Design review of the part built by this model. Coordinates are the model's own, in mm. A direction names the side the tool comes from. Coordinates: 2 decimals unless noted, no trailing zeros. Loops run counter-clockwise (first coordinate to the right, second up) from the corner with the lowest first, then second, coordinate; pieces in that order, holes last. Notation, with made-up numbers: M 45.5,87.5 L 55.5,87.5 A21 cw 55.5,116.5 Z; hole C 45.25,-16.75 d10. An arc over 180 degrees is marked long. Put each result on its own line as item: value. Start each with the question number.
(1) The part is to be moulded in two halves that separate along Z. For faces 4 (the flat face through (0, 0, -25)), 5 (the flat face through (-3, 12.5, 76)), 6 (the flat face through (-67, 0, 25)), say which applies: +Z half, -Z half, draft (parallel to the pull), parting line (faces both ways), or undercut.
(2) Take a section at D-D, the plane y = -27.5. Give the boundary of the cut face in (x, z).
(3) Take a section at A-A, the plane z = -100. Give the boundary of the cut face in (x, y).
(4) For probe 1 along Z at (x, y) = (69.5, 29); probe 2 along Y at (x, z) = (-16.5, 12); probe 3 along X at (y, z) = (13.5, -50), list the stretches that pass through material, from the lowest coordinate up. Write a range as [from, to].
(5) Clearance check with flat-ended pins moving along their axes: pin 1 (15 mm diameter, centred on y = 5.5, z = 9.5, fed in from +X); pin 2 (1.5 mm diameter, centred on x = -4, y = -8.5, fed in from -Z); pin 3 (12 mm diameter, centred on x = 3, z = 63, fed in from +Y). State where each tip first meets the part, or that it passes through.
(6) Take a section at B-B, the plane x = -65.5. Give the boundary of the cut face in (y, z).
(7) For faces 1 (the flat face through (-3, -22.5, -78)), 2 (the flat face through (67, 0, 25)), 3 (the flat face through (0, 0, 25)), list the 3-axis set-ups (+Z, -Z, +X, -X, +Y, -Y) from which the entire face can be reached by the end or side of a thin tool; tool diameter is ignored.
```python
from build123d import *

# Parameters (mm, degrees)
SKETCH1_W                = 175
SKETCH1_H                = 65
BOSS_EXTRUDE1_DEPTH      = 2
SKETCH2_W                = 175
SKETCH2_H                = 65
BOSS_EXTRUDE2_DEPTH      = 2
BOSS_EXTRUDE3_DEPTH      = 127
BOSS_EXTRUDE3_DEPTH_BACK = 127
SKETCH3_W                = 40
SKETCH3_H                = 4
BOSS_EXTRUDE4_DEPTH      = 2
BOSS_EXTRUDE5_DEPTH      = 2


with BuildPart() as part:
    # Sketch1 → Boss-Extrude1 (new body)
    with BuildSketch(Plane.XY.offset(25.0000008)):
        Rectangle(SKETCH1_W, SKETCH1_H)
    extrude(amount=BOSS_EXTRUDE1_DEPTH)



with BuildPart() as body_2:
    # Sketch2 → Boss-Extrude2 (new body)
    with BuildSketch(Plane.XY.offset(-25)):
        Rectangle(SKETCH2_W, SKETCH2_H)
    extrude(amount=-BOSS_EXTRUDE2_DEPTH)


with BuildPart() as part_1:
    add(part.part)

    add(body_2.part)  # Boss-Extrude3 merges body 2
    # Sketch3 → Boss-Extrude3 (add, two sides: drawn at the far end of the back side and taken through both)
    with BuildSketch(Plane.XY.offset(-BOSS_EXTRUDE3_DEPTH_BACK)):
        with Locations((-2.5, 14.5)):
            Rectangle(SKETCH3_W, SKETCH3_H)
        with Locations((-2.5, -20.5)):
            Rectangle(SKETCH3_W, SKETCH3_H)
    extrude(amount=BOSS_EXTRUDE3_DEPTH + BOSS_EXTRUDE3_DEPTH_BACK)

    # Sketch4 → Boss-Extrude4 (add)
    with BuildSketch(Plane(origin=(45.00000144, 0, 0), x_dir=(0, 0, -1), z_dir=(1, 0, 0))):
        Polygon((3.748957701, 32.5), (25, 32.5), (25, -32.5), (-25.0000008, -32.5), (-25.0000008, 32.5), (-3.748958501, 32.5), (-3.748958501, 25.45800753), (3.748957701, 25.45800753), align=None)
    extrude(amount=BOSS_EXTRUDE4_DEPTH)

    # Sketch5 → Boss-Extrude5 (add)
    with BuildSketch(Plane(origin=(-45.00000144, 0, 0), x_dir=(0, 0, -1), z_dir=(1, 0, 0))):
        Polygon((-25.0000008, 32.5), (-25.0000008, -32.5), (25, -32.5), (25, 32.5), (3.748957701, 32.5), (3.748957701, 25.45800753), (-3.748958501, 25.45800753), (-3.748958501, 32.5), align=None)
    extrude(amount=BOSS_EXTRUDE5_DEPTH)


solid = part_1.part
```
Computed values:
1. face 4: undercut
1. face 5: draft
1. face 6: undercut
2. outline: M -87.5,-27 L 87.5,-27 L 87.5,-25 L 47,-25 L 47,25 L 87.5,25 L 87.5,27 L -87.5,27 L -87.5,25 L -45,25 L -45,-25 L -87.5,-25 Z; hole M -43,-25 L 45,-25 L 45,25 L -43,25 Z
3. outline: M -22.5,-22.5 L 17.5,-22.5 L 17.5,-18.5 L -22.5,-18.5 Z; M -22.5,12.5 L 17.5,12.5 L 17.5,16.5 L -22.5,16.5 Z
4. probe 1: z = [-27, -25], [25, 27]
4. probe 2: y = [-22.5, -18.5], [12.5, 16.5]
4. probe 3: x = [-22.5, 17.5]
5. pin 1: stops at x = 47
5. pin 2: stops at z = -27
5. pin 3: stops at y = 16.5
6. outline: M -32.5,-27 L 32.5,-27 L 32.5,-25 L -32.5,-25 Z; M -32.5,25 L 32.5,25 L 32.5,27 L -32.5,27 Z
7. face 1: -Z, +X, -X, -Y
7. face 2: +X, +Y, -Y
7. face 3: none
